from build123d import *

# Parameters (mm, degrees)
SKETCH1_W                                       = 44
SKETCH1_H                                       = 18
BOSS_EXTRUDE1_DEPTH                             = 2
CSK_FOR_M2_FLAT_HEAD_MACHINE_SCREW1_D           = 2.4
CSK_FOR_M2_FLAT_HEAD_MACHINE_SCREW1_DEPTH       = 10
CSK_FOR_M2_FLAT_HEAD_MACHINE_SCREW1_CSINK_D     = 4.4
CSK_FOR_M2_FLAT_HEAD_MACHINE_SCREW1_CSINK_ANGLE = 90
CSK_FOR_M2_FLAT_HEAD_MACHINE_SCREW1_TIP         = 0.721032743


with BuildPart() as part:
    # Sketch1 → Boss-Extrude1 (new body)
    with BuildSketch(Plane(origin=(0, 0, 0), x_dir=(1, 0, 0), z_dir=(0, 1, 0))):
        Rectangle(SKETCH1_W, SKETCH1_H)
    extrude(amount=BOSS_EXTRUDE1_DEPTH)

    # CSK for M2 Flat Head Machine Screw1
    with Locations(Plane(origin=(0, 2, 0), x_dir=(1, 0, 0), z_dir=(0, 1, 0))):
        with Locations((-17, 6), (17, 6), (-17, -6), (17, -6)):
            CounterSinkHole(CSK_FOR_M2_FLAT_HEAD_MACHINE_SCREW1_D / 2, CSK_FOR_M2_FLAT_HEAD_MACHINE_SCREW1_CSINK_D / 2, depth=CSK_FOR_M2_FLAT_HEAD_MACHINE_SCREW1_DEPTH, counter_sink_angle=CSK_FOR_M2_FLAT_HEAD_MACHINE_SCREW1_CSINK_ANGLE)
            with Locations((0, 0, -(CSK_FOR_M2_FLAT_HEAD_MACHINE_SCREW1_DEPTH + CSK_FOR_M2_FLAT_HEAD_MACHINE_SCREW1_TIP / 2))):  # 118° drill point
                Cone(0, CSK_FOR_M2_FLAT_HEAD_MACHINE_SCREW1_D / 2, CSK_FOR_M2_FLAT_HEAD_MACHINE_SCREW1_TIP, mode=Mode.SUBTRACT)


solid = part.part
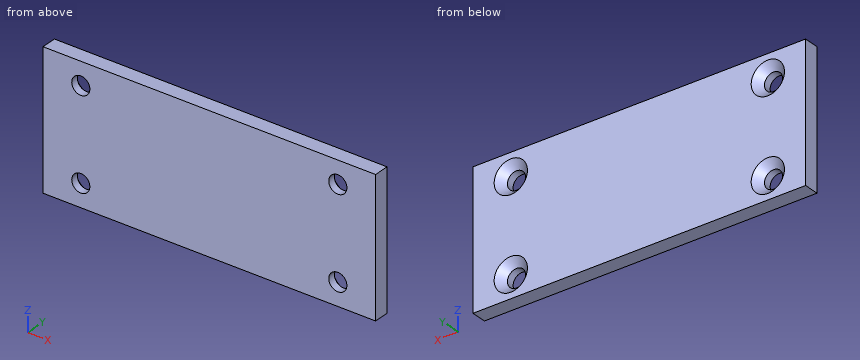
Check sheet for the modelled part. Datum: model origin and axes. Units: mm. Give positions to 0.01 mm unless a question says otherwise; leave off trailing zeros. Loops run counter-clockwise (first coordinate to the right, second up) from the corner with the lowest first, then second, coordinate; pieces in that order, holes last. Notation, with made-up numbers: M -39,9 L 2,9 A12 cw 2,24 Z; hole C 45,-19 d4. An arc over 180 degrees is marked long. Return JSON: item names as keys, results as strings. Group by question number.
1. Cross-section at A-A on z = -6. Record the boundary of the cut face in (x, y), plus the area to 3 significant figures.
2. Cross-section at C-C on x = -17. Record the boundary of the cut face in (y, z), plus the area to 3 significant figures.
3. Thickness scan on L1, parallel to X at y = 0.8, z = 6; L2, parallel to Z at x = -17, y = 0.8; L3, parallel to Z at x = -16.5, y = 1.4. Record the ranges inside material, lowest first.
4. Cross-section at B-B on y = 0.6. Record the boundary of the cut face in (x, z), plus the area to 3 significant figures.
5. Go/stop test with flat-tipped pins: pin 1 (3 mm diameter, centred on x = -17, z = -6, fed in from +Y); pin 2 (1.9 mm diameter, centred on x = -17, z = 6, fed in from +Y). Record where each tip stops, or that it passes through.
Return value:
{
 "1": {"outline": "M -22,0 L -18.2,0 L -18.2,1 L -19.2,2 L -22,2 Z; M -15.8,0 L 15.8,0 L 15.8,1 L 14.8,2 L -14.8,2 L -15.8,1 Z; M 18.2,0 L 22,0 L 22,2 L 19.2,2 L 18.2,1 Z", "area": "76.4 mm^2"},
 "2": {"outline": "M 0,-9 L 2,-9 L 2,-8.2 L 1,-7.2 L 0,-7.2 Z; M 0,-4.8 L 1,-4.8 L 2,-3.8 L 2,3.8 L 1,4.8 L 0,4.8 Z; M 0,7.2 L 1,7.2 L 2,8.2 L 2,9 L 0,9 Z", "area": "24.4 mm^2"},
 "3": {"L1": "-22 to -18.2, -15.8 to 15.8, 18.2 to 22", "L2": "-9 to -7.2, -4.8 to 4.8, 7.2 to 9", "L3": "-9 to -7.52, -4.48 to 4.48, 7.52 to 9"},
 "4": {"outline": "M -22,-9 L 22,-9 L 22,9 L -22,9 Z; hole C -17,-6 d2.4; hole C -17,6 d2.4; hole C 17,-6 d2.4; hole C 17,6 d2.4", "area": "774 mm^2"},
 "5": {"pin 1": "y = 1.3", "pin 2": "through"}
}
